Could you check a few things on this drawing? It's one solid part, dimensions in mm from its lowest x, y, z. A direction names the side the tool comes from. Round coordinates to 2 decimals unless told otherwise and drop trailing zeros. Loops run counter-clockwise (first coordinate to the right, second up) from the corner with the lowest first, then second, coordinate; pieces in that order, holes last. Notation, with made-up numbers: M 88.25,67 L 101.25,67 A11 cw 101.25,76 Z; hole C 15,-5.5 d9. An arc over 180 degrees is marked long. Write each question's results on one line, items separated by ' | '. Start each with the question number.
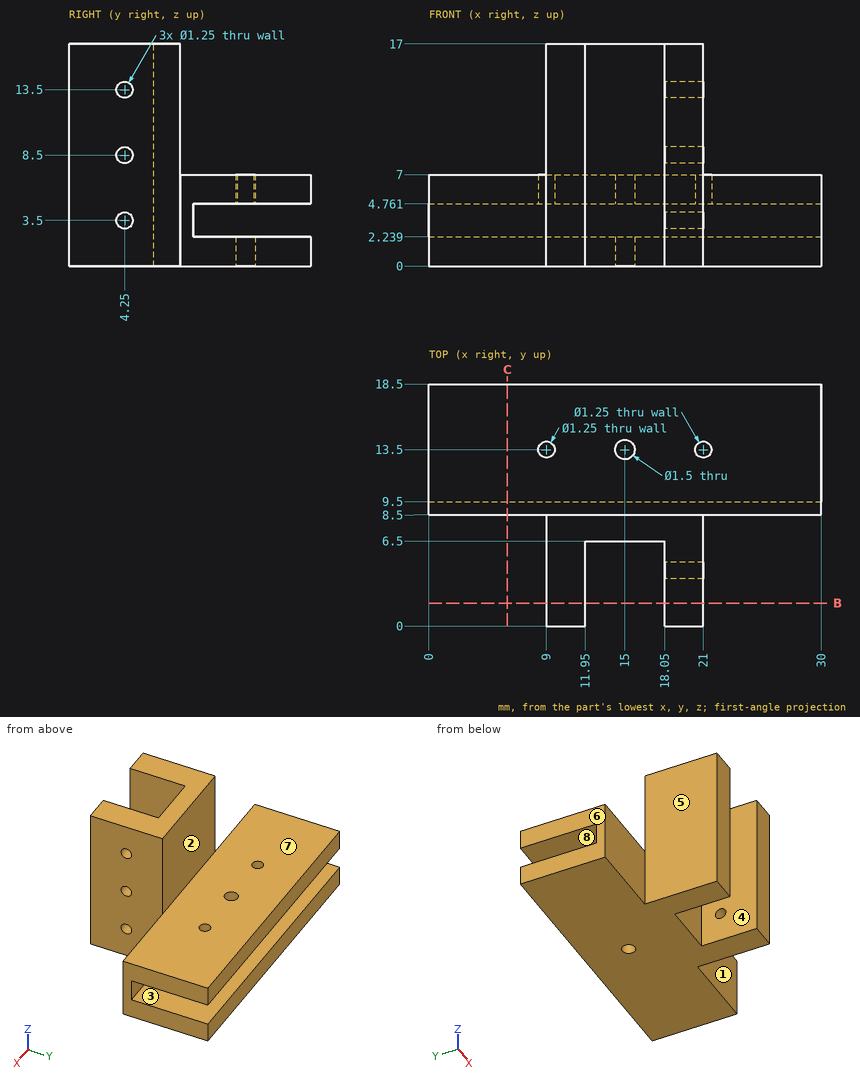
1. I want a section at B-B on y = 1.75. List the corners of the cut face in (x, z) for me, plus the area to 3 significant figures.
2. I want a section at C-C on x = 6. List the corners of the cut face in (y, z) for me.
3. I need wall thicknesses on line 1 along Z through (x, y) = (8, 12.5); line 2 along X through (y, z) = (2.5, 8.25); line 3 along Y through (x, z) = (18.8, 8.5) (1 decimal). Which ranges of each line are inside material? Lowest first, please.
4. Which directions (+Z, -Z, +X, -X, +Y, -Y) give clear straight access to the entire face, cutting with the end or side of a thin tool? Please do the marked faces 1, 2, 3, 4 and 5.
5. For pin 1 (2 mm diameter, centred on y = 4.25, z = 13.5, fed in from +X); pin 2 (2 mm diameter, centred on x = 5.5, z = 3.5, fed in from -Y); pin 3 (0.8 mm diameter, centred on x = 21, y = 13.5, fed in from +Z), each with a flat end and sliding along its axis, tell me the tip position at first contact or that it passes through.
6. If we mould it in two halves opening along Z, with no side actions, what happens to the marked faces 6, 7 and 8? For each: released by +Z, released by -Z, zero draft, split by the parting line, or undercut.
Outcome:
1) outline: M 9,0 L 11.95,0 L 11.95,17 L 9,17 Z; M 18.05,0 L 21,0 L 21,17 L 18.05,17 Z | area: 100 mm2
2) outline: M 8.5,0 L 18.5,0 L 18.5,2.24 L 9.5,2.24 L 9.5,4.76 L 18.5,4.76 L 18.5,7 L 8.5,7 Z
3) line 1: 0 to 2.24, 4.76 to 7 | line 2: 9 to 11.95, 18.05 to 21 | line 3: 0 to 3.6, 4.9 to 8.5
4) face 1: +Z, -Z, +X, -Y | face 2: +Z, +X, -X, +Y | face 3: +X, -X, +Y | face 4: +Z, -Z, -Y | face 5: +Z, -Z, -X, -Y
5) pin 1: x = 21 | pin 2: y = 8.5 | pin 3: z = 2.24
6) face 6: zero draft | face 7: released by +Z | face 8: undercut
